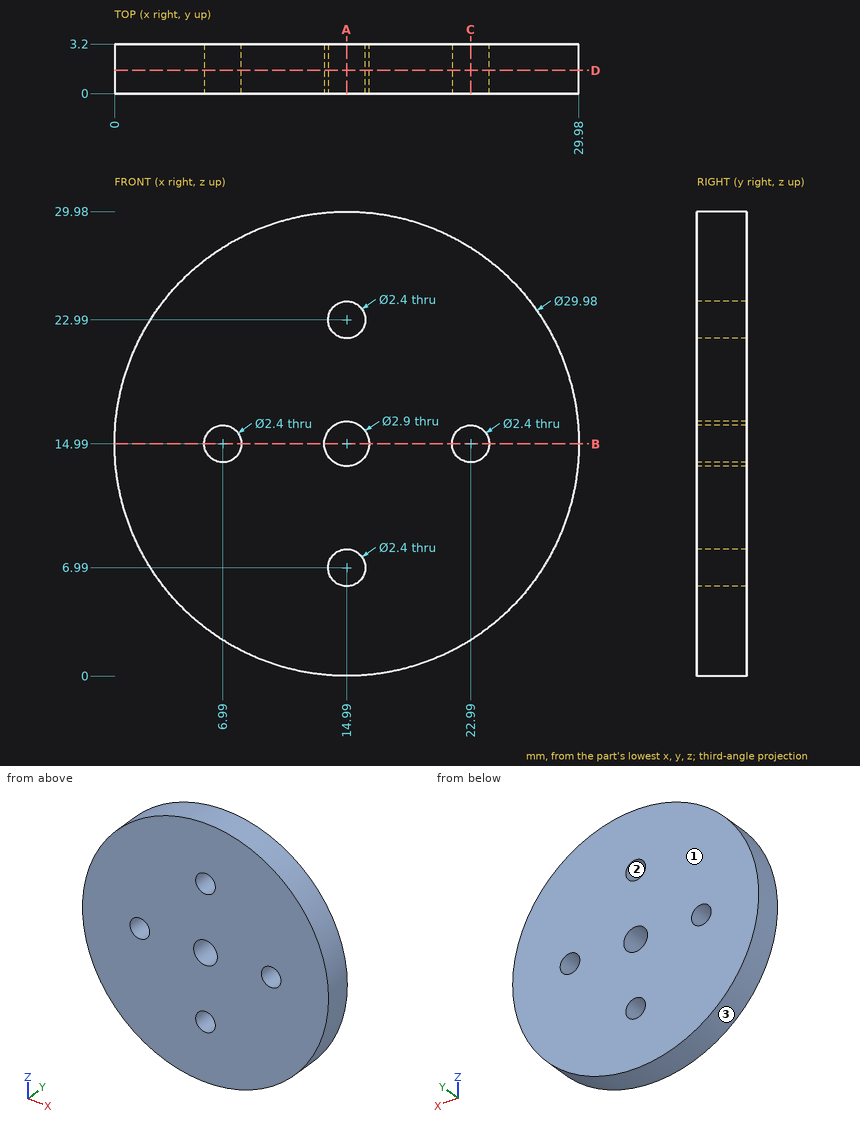
Design review of the part shown in the three views and the two pictorial views. Dimensions are in mm from the part's minimum x, y and z. Coordinates: 2 decimals unless noted, no trailing zeros. Loops run counter-clockwise (first coordinate to the right, second up) from the corner with the lowest first, then second, coordinate; pieces in that order, holes last. Notation, with made-up numbers: (-26, 83.5) - (6, 83.5) arc R31 cw to (6, 113.5) - close; hole circle Ø4 at (-28.75, -32.75). An arc over 180 degrees is marked (long way). Use a Markdown table: item, result. Add a question column.
Item 1: We need section A-A (x = 14.99). Give the boundary of the cut face in (y, z).
Item 2: We need section B-B (z = 14.99). Give the boundary of the cut face in (x, y).
Item 3: Insertion check: pin 1 Ø1.9 at (x, z) = (22.99, 14.99) entering from -Y; pin 2 Ø1 at (y, z) = (1, 7) entering from +X; pin 3 Ø1.5 at (y, z) = (0.5, 7) entering from -X. Each pin has a flat end and moves straight along its axis. Give the tip position at first contact, or say it passes through.
Item 4: We need section D-D (y = 1.5). Give the boundary of the cut face in (x, z), and give its area (3 significant figures).
Item 5: We need section C-C (x = 22.99). Give the boundary of the cut face in (y, z), and give its area (3 significant figures).
Item 6: Mouldability with a two-part tool opening along Z and no side actions: class the marked faces 1, 2 and 3 as pulls with the +Z half, pulls with the -Z half, needs draft (parallel to the pull), parting line crosses it, or undercut.
Item 7: For line 1 (X direction, y = 0.9, z = 14.99); line 2 (Z direction, x = 15.25, y = 1.2); line 3 (Z direction, x = 23.25, y = 2.75), list the stretches that pass through material, from the lowest coordinate up.
Results list:
| question | item | result |
|---|---|---|
| 1 | outline | (0, 0) - (3.2, 0) - (3.2, 5.79) - (0, 5.79) - close; (0, 8.19) - (3.2, 8.19) - (3.2, 13.54) - (0, 13.54) - close; (0, 16.44) - (3.2, 16.44) - (3.2, 21.79) - (0, 21.79) - close; (0, 24.19) - (3.2, 24.19) - (3.2, 29.98) - (0, 29.98) - close |
| 2 | outline | (0, 0) - (5.79, 0) - (5.79, 3.2) - (0, 3.2) - close; (8.19, 0) - (13.54, 0) - (13.54, 3.2) - (8.19, 3.2) - close; (16.44, 0) - (21.79, 0) - (21.79, 3.2) - (16.44, 3.2) - close; (24.19, 0) - (29.98, 0) - (29.98, 3.2) - (24.19, 3.2) - close |
| 3 | pin 1 | passes through |
| 3 | pin 2 | stops at x = 27.97 |
| 3 | pin 3 | stops at x = 1.86 |
| 4 | outline | circle Ø29.98 at (14.99, 14.99); hole circle Ø2.4 at (6.99, 14.99); hole circle Ø2.9 at (14.99, 14.99); hole circle Ø2.4 at (14.99, 6.99); hole circle Ø2.4 at (14.99, 22.99); hole circle Ø2.4 at (22.99, 14.99) |
| 4 | area | 681 mm^2 |
| 5 | outline | (0, 2.31) - (3.2, 2.31) - (3.2, 13.79) - (0, 13.79) - close; (0, 16.19) - (3.2, 16.19) - (3.2, 27.67) - (0, 27.67) - close |
| 5 | area | 73.5 mm^2 |
| 6 | face 1 | needs draft |
| 6 | face 2 | undercut |
| 6 | face 3 | parting line crosses it |
| 7 | line 1 | x = 0 to 5.79, 8.19 to 13.54, 16.44 to 21.79, 24.19 to 29.98 |
| 7 | line 2 | z = 0 to 5.82, 8.16 to 13.56, 16.42 to 21.82, 24.16 to 29.98 |
| 7 | line 3 | z = 2.48 to 13.82, 16.16 to 27.5 |
